Verification items for the finished model (mm, model axes). A direction names the side the tool comes from. Coordinates: 2 decimals unless noted, no trailing zeros. Order: outer loops, then holes, each group sorted by start corner. A loop starts at its lowest first (then second) coordinate and runs counter-clockwise, first axis right, second up. Notation, with made-up numbers: (-12.75, 20) -> (12.25, 20) arc R26 ccw to (12.25, 48) -> close; hole circle Ø10 at (67.5, -37). An arc over 180 degrees is marked (long way). Write item = value, one per line. Start each with the question number.
1. Cross-section at B-B on x = -6.25. Record the cut outline in (y, z), plus the area to 3 significant figures.
2. Cross-section at A-A on z = -1.75. Record the cut outline in (x, y), plus the area to 3 significant figures.
3. Go/stop test with flat-tipped pins: P1, Ø1, axis at x = 3, z = 3, coming from the +Y side; P2, Ø5, axis at x = -5, z = -2.5, coming from the +Y side. Record where each tip stops, or that it passes through.
4. Cross-section at C-C on y = 5.5. Record the cut outline in (x, z), plus the area to 3 significant figures.
5. Set-up check for faces 1 (the flat face through (0, 3, 5.08)), 2 (the flat face through (-5, 5.016, 0)): record each of +Z, -Z, +X, -X, +Y, -Y from which the full face is reachable in a straight line by a thin tool's end or side.
6. Thickness scan on line 1 along Y through (x, z) = (-4.75, -3.25); line 2 along X through (y, z) = (8.5, -4.25); line 3 along Y through (x, z) = (9, -4). Record the ranges inside material, lowest first. Write a range as from..to.
from build123d import *

# Parameters (mm, degrees)
SKETCH1_W           = 20.066
SKETCH1_H           = 10.033
BOSS_EXTRUDE1_DEPTH = 5.08
FILLET1_R           = 0.254
FILLET2_R           = 0.127


with BuildPart() as part:
    # Sketch1 → Boss-Extrude1 (new body, symmetric)
    with BuildSketch(Plane.XY):
        Polygon((-0.381, 5.0165), (10.033, 5.0165), (10.033, 9.0805), (4.826, 14.2875), (-0.381, 9.0805), align=None)
        Rectangle(SKETCH1_W, SKETCH1_H)
    extrude(amount=BOSS_EXTRUDE1_DEPTH, both=True)

    # Fillet1
    fillet1_edges = [part.edges().sort_by_distance(p)[0] for p in [
        (10.033, 9.0805, 0),
        (-0.381, 9.0805, 0),
    ]]
    fillet(fillet1_edges, radius=FILLET1_R)

    # Fillet2
    fillet2_edges = [part.edges().sort_by_distance(p)[0] for p in [
        (4.826, 14.2875, 0),
    ]]
    fillet(fillet2_edges, radius=FILLET2_R)


solid = part.part
Worked out:
q1.outline = (-5.02, -5.08) -> (5.02, -5.08) -> (5.02, 5.08) -> (-5.02, 5.08) -> close
q1.area = 102 mm²
q2.outline = (-10.03, -5.02) -> (10.03, -5.02) -> (10.03, 8.98) arc R0.25 ccw to (9.96, 9.15) -> (4.92, 14.2) arc R0.13 ccw to (4.74, 14.2) -> (-0.31, 9.15) arc R0.25 ccw to (-0.38, 8.98) -> (-0.38, 5.02) -> (-10.03, 5.02) -> close
q2.area = 271 mm²
q3.P1 = 12.96
q3.P2 = 5.02
q4.outline = (-0.38, -5.08) -> (10.03, -5.08) -> (10.03, 5.08) -> (-0.38, 5.08) -> close
q4.area = 106 mm²
q5.face_1 = +Z, +X, -X, +Y, -Y
q5.face_2 = +Z, -Z, -X, +Y
q6.line_1 = -5.02..5.02
q6.line_2 = -0.38..10.03
q6.line_3 = -5.02..10.11
